The listing builds one solid part. Answer for the finished solid, in the listing's coordinates (mm). A direction names the side the tool comes from. Give positions to 0.01 mm unless a question says otherwise; leave off trailing zeros. Loops run counter-clockwise (first coordinate to the right, second up) from the corner with the lowest first, then second, coordinate; pieces in that order, holes last. Notation, with made-up numbers: M -2,46.5 L 48,46.5 A27 ccw 48,65.5 Z; hole C -34.5,54.5 d10. An arc over 180 degrees is marked long. Return JSON: item names as keys, results as strings.
from build123d import *

# Parameters (mm, degrees)
F1_DEPTH = 1341.467
F2_R     = 5
F3_DEPTH = 50.801


with BuildPart() as f1:
    # F0 (on Front) → F1 (new body)
    with BuildSketch(Plane.XZ):
        with BuildLine():
            Line((-1.995114, 38.239733), (-40.095114, 38.239733))
            ThreePointArc((-40.095114, 38.239733), (-44.585242, 36.379861), (-46.445114, 31.889733))
            Line((-46.445114, 31.889733), (-46.445114, -31.610267))
            ThreePointArc((-46.445114, -31.610267), (-44.585242, -36.100395), (-40.095114, -37.960267))
            Line((-40.095114, -37.960267), (-1.995114, -37.960267))
            ThreePointArc((-1.995114, -37.960267), (2.495014, -36.100395), (4.354886, -31.610267))
            Line((4.354886, -31.610267), (4.354886, 31.889733))
            ThreePointArc((4.354886, 31.889733), (2.495014, 36.379861), (-1.995114, 38.239733))
        make_face()
        with BuildLine():
            ThreePointArc((-40.095114, 25.539733), (-38.235242, 30.029861), (-33.745114, 31.889733))
            Line((-33.745114, 31.889733), (-8.345114, 31.889733))
            ThreePointArc((-8.345114, 31.889733), (-3.854986, 30.029861), (-1.995114, 25.539733))
            Line((-1.995114, 25.539733), (-1.995114, -25.260267))
            ThreePointArc((-1.995114, -25.260267), (-3.854986, -29.750395), (-8.345114, -31.610267))
            Line((-8.345114, -31.610267), (-33.745114, -31.610267))
            ThreePointArc((-33.745114, -31.610267), (-38.235242, -29.750395), (-40.095114, -25.260267))
            Line((-40.095114, -25.260267), (-40.095114, 25.539733))
        make_face(mode=Mode.SUBTRACT)
    extrude(amount=F1_DEPTH)

    # F2 (on face) → F3 (cut, through all)
    with BuildSketch(Plane.YZ.offset(4.354886)):
        with Locations((-76.2, 15.139733)):
            Circle(F2_R)
        with Locations((-76.2, -14.860267)):
            Circle(F2_R)
        with Locations((-1265.267, -14.860267)):
            Circle(F2_R)
        with Locations((-1265.267, 15.139733)):
            Circle(F2_R)
    extrude(amount=-F3_DEPTH, mode=Mode.SUBTRACT)


solid = f1.part
(1) The part is cut by section A-A (y = -1032.5). Determine the outline of the cut face in (x, z), and give its area (3 significant figures).
Values follow:
{"outline": "M -46.45,-31.61 A6.35 ccw -40.1,-37.96 L -2,-37.96 A6.35 ccw 4.35,-31.61 L 4.35,31.89 A6.35 ccw -2,38.24 L -40.1,38.24 A6.35 ccw -46.45,31.89 Z; hole M -40.1,-25.26 A6.35 ccw -33.75,-31.61 L -8.35,-31.61 A6.35 ccw -2,-25.26 L -2,25.54 A6.35 ccw -8.35,31.89 L -33.75,31.89 A6.35 ccw -40.1,25.54 Z", "area": "1,450 mm²"}
(2) Straight lines are drawn through the part: line 1 along Z through (x, y) = (-0.25, -76.2); line 2 along X through (y, z) = (-859, -20.5); line 3 along Z through (x, y) = (-9.5, -1052). For each, find the intervals that lie inside material, in ascending order.
Values follow:
{"line 1": "-37.72 to -19.86, -9.86 to 10.14, 20.14 to 38", "line 2": "-46.45 to -40.1, -2 to 4.35", "line 3": "-37.96 to -31.61, 31.89 to 38.24"}
(3) Given pin 1 (9 mm diameter, centred on y = -1265.27, z = -14.86, fed in from +X); pin 2 (11.5 mm diameter, centred on y = -76.2, z = 15.14, fed in from +X), each flat-ended and moving along its own axis, determine where each tip first touches the part or whether it passes through.
Values follow:
{"pin 1": "through", "pin 2": "x = 4.35"}
(4) Determine the mould class of faces 3 (the flat face through (-21, -661, -37.96)), 4 (the flat face through (-46.445, -661, 1)), 5 (the flat face through (-21, -661, 38.24)), 6 (the flat face through (-1.995, -661, 0)) for opening direction Z: released by +Z, released by -Z, zero draft, split by the parting line, or undercut.
Values follow:
{"face 3": "released by -Z", "face 4": "zero draft", "face 5": "released by +Z", "face 6": "undercut"}
(5) The part is cut by section B-B (x = -25.5). Determine the outline of the cut face in (y, z).
Values follow:
{"outline": "M -1341.47,-37.96 L 0,-37.96 L 0,-31.61 L -1341.47,-31.61 Z; M -1341.47,31.89 L 0,31.89 L 0,38.24 L -1341.47,38.24 Z"}
(6) A tool of negligible diameter and unlimited length cuts with its end or side. For faces 1 (the flat face through (-44, -1341.467, 1)), 2 (the flat face through (-21, -661, 31.89)), from which of +Z, -Z, +X, -X, +Y, -Y can it reach the whole face along a straight path? Write none if from no direction.
Values follow:
{"face 1": "+Z, -Z, +X, -X, -Y", "face 2": "+Y, -Y"}
